Check sheet for the modelled part. Datum: model origin and axes. Units: mm. A direction names the side the tool comes from. Coordinates: 2 decimals unless noted, no trailing zeros. Write each loop counter-clockwise with the first axis right and the second up, starting at its lowest first coordinate (ties: lowest second). Pieces come first, ordered by that corner, then holes. Notation, with made-up numbers: (12, 42.25) -> (70, 42.25) arc R23 cw to (70, 56.25) -> close; hole circle Ø7 at (31, 88.5). An arc over 180 degrees is marked (long way). Put each result on its own line as item: value.
```python
from build123d import *

# Parameters (mm, degrees)
SKETCH_1_W          = 50
SKETCH_1_H          = 20
SKETCH_1_R          = 2.65
EXTRUDE_1_DEPTH     = 15
SKETCH_2_R          = 5.175
CUT_EXTRUDE_1_DEPTH = 5.5
SKETCH_3_R          = 8.15
CUT_EXTRUDE_2_DEPTH = 4.8
EXTRUDE_2_DEPTH     = 10
SKETCH_5_R          = 8.2
CUT_EXTRUDE_3_DEPTH = 6
CUT_EXTRUDE_4_DEPTH = 63.24949799
FILLET_1_R          = 1
FILLET_3_R          = 10


with BuildPart() as part:
    # 草图1 → 凸台-拉伸1 (new body)
    with BuildSketch(Plane.XY):
        Rectangle(SKETCH_1_W, SKETCH_1_H)
        with Locations((-18.5, 0)):
            Circle(SKETCH_1_R, mode=Mode.SUBTRACT)
        with Locations((18.5, 0)):
            Circle(SKETCH_1_R, mode=Mode.SUBTRACT)
    extrude(amount=EXTRUDE_1_DEPTH)

    # 草图2 → 切除-拉伸1 (cut)
    with BuildSketch(Plane(origin=(0, 0, 0), x_dir=(-1, 0, 0), z_dir=(0, 0, -1))):
        Circle(SKETCH_2_R)
    extrude(amount=-CUT_EXTRUDE_1_DEPTH, mode=Mode.SUBTRACT)

    # 草图3 → 切除-拉伸2 (cut)
    with BuildSketch(Plane.XY.offset(15)):
        Circle(SKETCH_3_R)
    extrude(amount=-CUT_EXTRUDE_2_DEPTH, mode=Mode.SUBTRACT)

    # 草图4 → 凸台-拉伸2 (add)
    with BuildSketch(Plane(origin=(0, 0, 0), x_dir=(-1, 0, 0), z_dir=(0, 0, -1))):
        with BuildLine():
            Line((25, 10), (9.265702954, 48.761216396))
            ThreePointArc((9.265702954, 48.761216396), (0, 55), (-9.265702954, 48.761216396))
            Line((-9.265702954, 48.761216396), (-25, 10))
            Line((-25, 10), (25, 10))
        make_face()
    extrude(amount=-EXTRUDE_2_DEPTH)

    # 草图5 → 切除-拉伸3 (cut)
    with BuildSketch(Plane(origin=(0, 0, 0), x_dir=(-1, 0, 0), z_dir=(0, 0, -1))):
        with Locations((0, 45)):
            Circle(SKETCH_5_R)
    extrude(amount=-CUT_EXTRUDE_3_DEPTH, mode=Mode.SUBTRACT)

    # 草图6 → 切除-拉伸4 (cut, through all)
    with BuildSketch(Plane(origin=(0, 0, 0), x_dir=(-1, 0, 0), z_dir=(0, 0, -1))):
        Polygon((-20.683004279, 10), (-5, 48.634857396), (-5, 10), align=None)
        Polygon((5, 10), (20.683004279, 10), (5, 48.634857396), align=None)
    extrude(amount=-CUT_EXTRUDE_4_DEPTH, mode=Mode.SUBTRACT)

    # 圆角1
    fillet_1_edges = [part.edges().sort_by_distance(p)[0] for p in [
        (5, 10, 5),
        (20.683004279, 10, 5),
        (5, 48.634857396, 8),
        (-20.683004279, 10, 5),
        (-5, 10, 5),
        (-5, 48.634857396, 8),
    ]]
    fillet(fillet_1_edges, radius=FILLET_1_R)

    # 圆角3
    fillet_3_edges = [part.edges().sort_by_distance(p)[0] for p in [
        (25, -10, 7.5),
        (-25, -10, 7.5),
    ]]
    fillet(fillet_3_edges, radius=FILLET_3_R)


solid = part.part
```
Q1. Cross-section at B-B (x = 0). Record the cut outline in (y, z) (3 decimals), plus the area to 3 significant figures.
Recorded:
outline: (-10, 0) -> (-5.175, 0) -> (-5.175, 5.5) -> (5.175, 5.5) -> (5.175, 0) -> (36.8, 0) -> (36.8, 6) -> (53.2, 6) -> (53.2, 0) -> (55, 0) -> (55, 10) -> (10, 10) -> (10, 15) -> (8.15, 15) -> (8.15, 10.2) -> (-8.15, 10.2) -> (-8.15, 15) -> (-10, 15) -> close
area: 516 mm2
Q2. Tool access check on faces 5 (the cylindrical face through (20.035, 10.453, 5.07)), 6 (the cylindrical face through (4.107, -3.149, 2.712)), 7 (the cylindrical face through (-6.468, -4.959, 12.634)). Record the directions out of +Z, -Z, +X, -X, +Y, -Y that give a thin tool (end or side, any length) a straight path to the whole face; none if there is none.
Recorded:
face 5: +Z, -Z
face 6: -Z
face 7: +Z
Q3. Material ranges on line 1 along Y through (x, z) = (2, 4.5); line 2 along Y through (x, z) = (18.5, 6.75); line 3 along X through (y, z) = (30, 5), recorded low to high.
Recorded:
line 1: y = -10 to -4.77, 4.77 to 37.05, 52.95 to 54.8
line 2: y = -9.37 to -2.65, 2.65 to 10, 15.38 to 26.01
line 3: x = -16.88 to -12.56, -5 to 5, 12.56 to 16.88
Q4. Cross-section at C-C (x = -18.5). Record the cut outline in (y, z), plus the area to 3 significant figures.
Recorded:
outline: (-9.37, 0) -> (-2.65, 0) -> (-2.65, 15) -> (-9.37, 15) -> close; (2.65, 0) -> (10, 0) -> (10, 15) -> (2.65, 15) -> close; (15.38, 0) -> (26.01, 0) -> (26.01, 10) -> (15.38, 10) -> close
area: 317 mm2
Q5. Depth check by flat-ended pin: P1, Ø2, axis at y = 23.5, z = 9.5, coming from the +X side; P2, Ø5, axis at y = 34, z = 4.5, coming from the +X side; P3, Ø5, axis at x = 2, y = 46.5, coming from the -Z side. Enter the tip coordinate at first touch or a pass-through.
Recorded:
P1: stops at x = 19.93
P2: stops at x = 16.27
P3: stops at z = 6
Q6. Cross-section at A-A (z = 7.25). Record the cut outline in (x, y).
Recorded:
outline: (-25, 0) arc R10 ccw to (-15, -10) -> (15, -10) arc R10 ccw to (25, 0) -> (25, 10) -> (9.27, 48.76) arc R10 ccw to (-9.27, 48.76) -> (-25, 10) -> close; hole circle Ø5.3 at (-18.5, 0); hole (-20.12, 11.38) arc R1 ccw to (-19.2, 10) -> (-6, 10) arc R1 ccw to (-5, 11) -> (-5, 43.51) arc R1 ccw to (-6.93, 43.89) -> close; hole (5, 11) arc R1 ccw to (6, 10) -> (19.2, 10) arc R1 ccw to (20.12, 11.38) -> (6.93, 43.89) arc R1 ccw to (5, 43.51) -> close; hole circle Ø5.3 at (18.5, 0)
Q7. Cross-section at D-D (y = 37.5). Record the cut outline in (x, z).
Recorded:
outline: (-13.84, 0) -> (-9.52, 0) -> (-9.52, 10) -> (-13.84, 10) -> close; (-5, 0) -> (-3.32, 0) -> (-3.32, 6) -> (3.32, 6) -> (3.32, 0) -> (5, 0) -> (5, 10) -> (-5, 10) -> close; (9.52, 0) -> (13.84, 0) -> (13.84, 10) -> (9.52, 10) -> close
Q8. Mould release check, pull along Y, two halves, no side actions. Record for faces 1 (the flat face through (-25, 5, 7)), 2 (the cylindrical face through (0.1, 36.8, 3)), 3 (the cylindrical face through (21.028, 0.796, 7.395)), 4 (the flat face through (0, -10, 7)): released by +Y, released by -Y, zero draft, split by the parting line, or undercut.
Recorded:
face 1: zero draft
face 2: undercut
face 3: undercut
face 4: released by -Y
